The model under review builds one solid part; all positions refer to its coordinate system, in mm. A direction names the side the tool comes from. Give positions to 0.01 mm unless a question says otherwise; leave off trailing zeros. Order: outer loops, then holes, each group sorted by start corner. A loop starts at its lowest first (then second) coordinate and runs counter-clockwise, first axis right, second up. Notation, with made-up numbers: (-10, 1.5) - (15, 1.5) arc R26 cw to (15, 24.5) - close; hole circle Ø8 at (-37, 68.5). An arc over 180 degrees is marked (long way). Write item = value, one per line. Start each with the question number.
1. Machinability: for faces 5 (the flat face through (1.5, -13.9, 18.5)), 6 (the flat face through (0, -6, 27)), 7 (the flat face through (-1.5, 13.8, 18.5)), 8 (the flat face through (2.9, 0, 25)), 9 (the flat face through (-0.5, -16, 17)), which of the approach directions +Z, -Z, +X, -X, +Y, -Y give a long, thin tool a straight path to every point of the face, cutting with its end or side? Answer none if there is none.
2. Mouldability with a two-part tool opening along X and no side actions: class faces 1 (the flat face through (6.25, 0, 11)), 2 (the flat face through (-3, -16.35, 17)), 3 (the cylindrical face through (-0.064, 3.164, 24.972)), 4 (the cylindrical face through (0, -13.9, 5.5)) as pulls with the +X half, pulls with the -X half, needs draft (parallel to the pull), parting line crosses it, or undercut.
3. For P1, Ø6, axis at x = -1.5, y = 4.5, coming from the +Z side; P2, Ø0.5, axis at y = 0, z = 24.5, coming from the +X side; P3, Ø1, axis at x = 0, z = 12, coming from the -Y side, all flat-tipped, find the tip position at first contact; note any pin that passes through.
4. We need section B-B, the plane y = -5.6. Give the boundary of the cut face in (x, z), and give its area (3 significant figures).
5. We need section D-D, the plane z = 12. Give the boundary of the cut face in (x, y).
6. Wall thickness on probe 1 along X at (y, z) = (-13.85, 16.8); probe 2 along Y at (x, z) = (0, 27.7); probe 3 along Z at (x, y) = (5, -12.5): over which ranges is each line inside the solid? List them lowest first.
7. We need section C-C, the plane x = 4. Give the boundary of the cut face in (y, z), and give its area (3 significant figures).
8. We need section A-A, the plane y = -13.85. Give the boundary of the cut face in (x, z) (3 decimals), and give its area (3 significant figures).
from build123d import *

# Parameters (mm, degrees)
SKETCH1_W           = 12.5
SKETCH1_H           = 22.7
BOSS_EXTRUDE1_DEPTH = 23
BOSS_EXTRUDE2_DEPTH = 4
SKETCH3_W           = 2.3
SKETCH3_H           = 5
BOSS_EXTRUDE3_DEPTH = 6.25
CUT_EXTRUDE1_REACH  = 20.5
BOSS_EXTRUDE4_START = -4
SKETCH5_W           = 4
SKETCH5_H           = 5
BOSS_EXTRUDE4_DEPTH = 1.5
SKETCH6_R           = 2.35
SKETCH6_R_2         = 0.8
BOSS_EXTRUDE5_DEPTH = 2.4
SKETCH7_W           = 4.514706964
SKETCH7_H           = 2.103718672
CUT_EXTRUDE2_DEPTH  = 5


with BuildPart() as part:
    # Sketch1 → Boss-Extrude1 (new body)
    with BuildSketch(Plane.XY):
        Rectangle(SKETCH1_W, SKETCH1_H)
    extrude(amount=BOSS_EXTRUDE1_DEPTH)

    # Sketch2 → Boss-Extrude2 (add)
    with BuildSketch(Plane.XY.offset(23)):
        with BuildLine():
            Line((2.9, 0.265128397), (2.9, -0.634871603))
            ThreePointArc((2.9, -0.634871603), (0, -11.35), (-2.9, -0.634871603))
            Line((-2.9, -0.634871603), (-2.9, 0.265128397))
            ThreePointArc((-2.9, 0.265128397), (0, 3.165128397), (2.9, 0.265128397))
        make_face()
    extrude(amount=BOSS_EXTRUDE2_DEPTH)

    # Sketch3 → Boss-Extrude3 (add, symmetric)
    with BuildSketch(Plane(origin=(0, 0, 0), x_dir=(0, 0, -1), z_dir=(1, 0, 0))):
        with Locations((-17.35, 13.85)):
            Rectangle(SKETCH3_W, SKETCH3_H)
        with Locations((-17.35, -13.85)):
            Rectangle(SKETCH3_W, SKETCH3_H)
    extrude(amount=BOSS_EXTRUDE3_DEPTH, both=True)

    # Sketch4 → Cut-Extrude1 (cut, up to next)
    with BuildSketch(Plane.XY.offset(18.5), mode=Mode.PRIVATE) as cut_extrude1_sk1:
        with BuildLine():
            Line((0.5, 16.35), (-0.5, 16.35))
            Line((-0.5, 16.35), (-0.5, 14.995643924))
            ThreePointArc((-0.5, 14.995643924), (0, 12.6), (0.5, 14.995643924))
            Line((0.5, 14.995643924), (0.5, 16.35))
        make_face()
    cut_extrude1_tool1 = extrude(cut_extrude1_sk1.sketch, amount=-CUT_EXTRUDE1_REACH, mode=Mode.PRIVATE) & part.part
    add(cut_extrude1_tool1.solids().sort_by_distance((0, 14.235184, 18.5))[0], mode=Mode.SUBTRACT)
    # Sketch4 → Cut-Extrude1 (cut, up to next)
    with BuildSketch(Plane.XY.offset(18.5), mode=Mode.PRIVATE) as cut_extrude1_sk2:
        with BuildLine():
            Line((-0.5, -16.35), (-0.5, -14.995643924))
            ThreePointArc((-0.5, -14.995643924), (0, -12.6), (0.5, -14.995643924))
            Line((0.5, -14.995643924), (0.5, -16.35))
            Line((0.5, -16.35), (-0.5, -16.35))
        make_face()
    cut_extrude1_tool2 = extrude(cut_extrude1_sk2.sketch, amount=-CUT_EXTRUDE1_REACH, mode=Mode.PRIVATE) & part.part
    add(cut_extrude1_tool2.solids().sort_by_distance((0, -14.235184, 18.5))[0], mode=Mode.SUBTRACT)

    # Sketch5 → Boss-Extrude4 (add)
    with BuildSketch(Plane(origin=(0, 0, 0), x_dir=(-1, 0, 0), z_dir=(0, 0, -1)).offset(BOSS_EXTRUDE4_START)):
        with Locations((0, -13.85)):
            Rectangle(SKETCH5_W, SKETCH5_H)
    extrude(amount=-BOSS_EXTRUDE4_DEPTH)

    # Sketch6 → Boss-Extrude5 (add)
    with BuildSketch(Plane.XY.offset(27)):
        with Locations((0, -5.6)):
            Circle(SKETCH6_R)
        with Locations((0, -5.6)):
            Circle(SKETCH6_R_2, mode=Mode.SUBTRACT)
    extrude(amount=BOSS_EXTRUDE5_DEPTH)

    # Sketch7 → Cut-Extrude2 (cut)
    with BuildSketch(Plane.XZ.offset(16.35)):
        with Locations((0, 4.75)):
            Rectangle(SKETCH7_W, SKETCH7_H)
        with BuildLine():
            ThreePointArc((-0.625, 4.335421901), (-2, 4.75), (-0.625, 5.164578099))
            ThreePointArc((-0.625, 5.164578099), (0, 5.5), (0.625, 5.164578099))
            ThreePointArc((0.625, 5.164578099), (2, 4.75), (0.625, 4.335421901))
            ThreePointArc((0.625, 4.335421901), (0, 4), (-0.625, 4.335421901))
        make_face(mode=Mode.SUBTRACT)
    extrude(amount=-CUT_EXTRUDE2_DEPTH, mode=Mode.SUBTRACT)


solid = part.part
Model answer:
q1.face_5 = +Z, +X, -X, -Y
q1.face_6 = +Z
q1.face_7 = +Z, +X, -X, +Y
q1.face_8 = +Z, +X, +Y
q1.face_9 = +Z, -Y
q2.face_1 = pulls with the +X half
q2.face_2 = needs draft
q2.face_3 = parting line crosses it
q2.face_4 = undercut
q3.P1 = 27
q3.P2 = 2.9
q3.P3 = -11.35
q4.outline = (-6.25, 0) - (6.25, 0) - (6.25, 23) - (5.75, 23) - (5.75, 27) - (2.35, 27) - (2.35, 29.4) - (0.8, 29.4) - (0.8, 27) - (-0.8, 27) - (-0.8, 29.4) - (-2.35, 29.4) - (-2.35, 27) - (-5.75, 27) - (-5.75, 23) - (-6.25, 23) - close
q4.area = 341 mm2
q5.outline = (-6.25, -11.35) - (6.25, -11.35) - (6.25, 11.35) - (-6.25, 11.35) - close
q6.probe_1 = -6.25 to -1.25, 1.25 to 6.25
q6.probe_2 = -7.95 to -6.4, -4.8 to -3.25
q6.probe_3 = 16.2 to 18.5
q7.outline = (-16.35, 16.2) - (-11.35, 16.2) - (-11.35, 0) - (11.35, 0) - (11.35, 16.2) - (16.35, 16.2) - (16.35, 18.5) - (11.35, 18.5) - (11.35, 23) - (-1.47, 23) - (-1.47, 27) - (-9.73, 27) - (-9.73, 23) - (-11.35, 23) - (-11.35, 18.5) - (-16.35, 18.5) - close
q7.area = 578 mm2
q8.outline = (-6.25, 16.2) - (-1.25, 16.2) - (-1.25, 18.5) - (-6.25, 18.5) - close; (-0.625, 4.335) arc R0.75 ccw to (0.625, 4.335) arc R0.75 ccw (long way) to (0.625, 5.165) arc R0.75 ccw to (-0.625, 5.165) arc R0.75 ccw (long way) to start; (1.25, 16.2) - (6.25, 16.2) - (6.25, 18.5) - (1.25, 18.5) - close
q8.area = 28.0 mm2
